```python
from build123d import *

# Parameters (mm, degrees)
SKETCH3_R           = 1.905
BOSS_EXTRUDE1_DEPTH = 6.35
CUT_EXTRUDE1_DEPTH  = 133.5410974
SKETCH5_R           = 1.905
BOSS_EXTRUDE2_DEPTH = 12.700000124
CUT_EXTRUDE2_START  = -6.350000124
SKETCH6_R           = 1.905
SKETCH6_R_2         = 1.75
CUT_EXTRUDE2_DEPTH  = 6.350000124


with BuildPart() as part:
    # Sketch3 → Boss-Extrude1 (new body)
    with BuildSketch(Plane(origin=(0, 0, 0), x_dir=(1, 0, 0), z_dir=(0, 1, 0))):
        Polygon((-19.05, -82.55), (-12.7, -88.9), (12.7, -88.9), (19.05, -82.55), (19.05, -74.93), (19.05, -68.58), (19.05, -60.96), (19.05, -38.1), (19.05, -30.48), (19.05, -24.13), (19.05, -16.51), (49.05, 15.745), (49.05, 27.745), (-49.05, 27.745), (-49.05, 15.745), (-19.05, -16.51), (-19.05, -24.13), (-19.05, -30.48), (-19.05, -38.1), (-19.05, -60.96), (-19.05, -68.58), (-19.05, -74.93), align=None)
        with Locations(Location((-15.24, -78.74, 0), (0, 0, 270))):
            Circle(SKETCH3_R, mode=Mode.SUBTRACT)
        with Locations(Location((15.24, -78.74, 0), (0, 0, 270))):
            Circle(SKETCH3_R, mode=Mode.SUBTRACT)
        with Locations(Location((15.24, -64.77, 0), (0, 0, 270))):
            Circle(SKETCH3_R, mode=Mode.SUBTRACT)
        with Locations(Location((-15.24, -64.77, 0), (0, 0, 270))):
            Circle(SKETCH3_R, mode=Mode.SUBTRACT)
        with Locations(Location((-15.24, -20.32, 0), (0, 0, 270))):
            Circle(SKETCH3_R, mode=Mode.SUBTRACT)
        with Locations(Location((15.24, -20.32, 0), (0, 0, 270))):
            Circle(SKETCH3_R, mode=Mode.SUBTRACT)
        with Locations(Location((15.24, -34.29, 0), (0, 0, 270))):
            Circle(SKETCH3_R, mode=Mode.SUBTRACT)
        with Locations(Location((-15.24, -34.29, 0), (0, 0, 270))):
            Circle(SKETCH3_R, mode=Mode.SUBTRACT)
    extrude(amount=BOSS_EXTRUDE1_DEPTH)

    # Sketch4 → Cut-Extrude1 (cut, through all)
    with BuildSketch(Plane.ZY.offset(49.05)):
        Polygon((-21.395, 0), (-27.745, 0), (-27.745, 5), align=None)
    extrude(amount=-CUT_EXTRUDE1_DEPTH, mode=Mode.SUBTRACT)

    # Sketch5 → Boss-Extrude2 (add)
    with BuildSketch(Plane.XZ):
        with Locations(Location((-15.24, 20.32, 0), (0, 0, 270))):
            Circle(SKETCH5_R)
        with Locations(Location((-15.24, 34.29, 0), (0, 0, 270))):
            Circle(SKETCH5_R)
        with Locations(Location((15.24, 20.32, 0), (0, 0, 270))):
            Circle(SKETCH5_R)
        with Locations(Location((15.24, 34.29, 0), (0, 0, 270))):
            Circle(SKETCH5_R)
        with Locations(Location((15.24, 64.77, 0), (0, 0, 270))):
            Circle(SKETCH5_R)
        with Locations(Location((15.24, 78.74, 0), (0, 0, 270))):
            Circle(SKETCH5_R)
        with Locations(Location((-15.24, 64.77, 0), (0, 0, 270))):
            Circle(SKETCH5_R)
        with Locations(Location((-15.24, 78.74, 0), (0, 0, 270))):
            Circle(SKETCH5_R)
    extrude(amount=-BOSS_EXTRUDE2_DEPTH)

    # Sketch6 → Cut-Extrude2 (cut)
    # profile 1 of 8: a face of its own
    with BuildSketch(Plane(origin=(0, 12.700000124, 0), x_dir=(1, 0, 0), z_dir=(0, 1, 0)).offset(CUT_EXTRUDE2_START)):
        with Locations((-15.24, -78.74)):
            Circle(SKETCH6_R)
        with Locations(Location((-15.24, -78.74, 0), (0, 0, 270))):
            Circle(SKETCH6_R_2, mode=Mode.SUBTRACT)
    # profile 2 of 8: a face of its own
    with BuildSketch(Plane(origin=(0, 12.700000124, 0), x_dir=(1, 0, 0), z_dir=(0, 1, 0)).offset(CUT_EXTRUDE2_START)):
        with Locations((15.24, -78.74)):
            Circle(SKETCH6_R)
        with Locations(Location((15.24, -78.74, 0), (0, 0, 270))):
            Circle(SKETCH6_R_2, mode=Mode.SUBTRACT)
    # profile 3 of 8: a face of its own
    with BuildSketch(Plane(origin=(0, 12.700000124, 0), x_dir=(1, 0, 0), z_dir=(0, 1, 0)).offset(CUT_EXTRUDE2_START)):
        with Locations((15.24, -64.77)):
            Circle(SKETCH6_R)
        with Locations(Location((15.24, -64.77, 0), (0, 0, 270))):
            Circle(SKETCH6_R_2, mode=Mode.SUBTRACT)
    # profile 4 of 8: a face of its own
    with BuildSketch(Plane(origin=(0, 12.700000124, 0), x_dir=(1, 0, 0), z_dir=(0, 1, 0)).offset(CUT_EXTRUDE2_START)):
        with Locations((-15.24, -64.77)):
            Circle(SKETCH6_R)
        with Locations(Location((-15.24, -64.77, 0), (0, 0, 270))):
            Circle(SKETCH6_R_2, mode=Mode.SUBTRACT)
    # profile 5 of 8: a face of its own
    with BuildSketch(Plane(origin=(0, 12.700000124, 0), x_dir=(1, 0, 0), z_dir=(0, 1, 0)).offset(CUT_EXTRUDE2_START)):
        with Locations((-15.24, -34.29)):
            Circle(SKETCH6_R)
        with Locations(Location((-15.24, -34.29, 0), (0, 0, 270))):
            Circle(SKETCH6_R_2, mode=Mode.SUBTRACT)
    # profile 6 of 8: a face of its own
    with BuildSketch(Plane(origin=(0, 12.700000124, 0), x_dir=(1, 0, 0), z_dir=(0, 1, 0)).offset(CUT_EXTRUDE2_START)):
        with Locations((15.24, -34.29)):
            Circle(SKETCH6_R)
        with Locations(Location((15.24, -34.29, 0), (0, 0, 270))):
            Circle(SKETCH6_R_2, mode=Mode.SUBTRACT)
    # profile 7 of 8: a face of its own
    with BuildSketch(Plane(origin=(0, 12.700000124, 0), x_dir=(1, 0, 0), z_dir=(0, 1, 0)).offset(CUT_EXTRUDE2_START)):
        with Locations((15.24, -20.32)):
            Circle(SKETCH6_R)
        with Locations(Location((15.24, -20.32, 0), (0, 0, 270))):
            Circle(SKETCH6_R_2, mode=Mode.SUBTRACT)
    # profile 8 of 8: a face of its own
    with BuildSketch(Plane(origin=(0, 12.700000124, 0), x_dir=(1, 0, 0), z_dir=(0, 1, 0)).offset(CUT_EXTRUDE2_START)):
        with Locations((-15.24, -20.32)):
            Circle(SKETCH6_R)
        with Locations(Location((-15.24, -20.32, 0), (0, 0, 270))):
            Circle(SKETCH6_R_2, mode=Mode.SUBTRACT)
    extrude(amount=CUT_EXTRUDE2_DEPTH, mode=Mode.SUBTRACT)


solid = part.part
```
For this review, take the finished solid that the model builds, in its own axes (mm). A direction names the side the tool comes from. Round coordinates to 2 decimals unless told otherwise and drop trailing zeros. Order: outer loops, then holes, each group sorted by start corner. A loop starts at its lowest first (then second) coordinate and runs counter-clockwise, first axis right, second up. Notation, with made-up numbers: (0, -26.5) -> (18, -26.5) arc R26 cw to (18, 3.5) -> close; hole circle Ø6 at (-38.5, -26.5). An arc over 180 degrees is marked (long way). Use a Markdown table: item, result.
Item 1: Draft analysis for pull direction X (two halves, no side actions). For faces 1 (the flat face through (-49.05, 4, -20)), 2 (the cylindrical face through (-15.16, 9.48, 76.99)), 3 (the flat face through (15, 12.7, 20)), state which applies: +X half, -X half, draft (parallel to the pull), parting line (faces both ways), or undercut.
Resolved:
| item | result |
|---|---|
| face 1 | -X half |
| face 2 | undercut |
| face 3 | draft |
Item 2: Take a section at D-D (z = 45). State the section outline as (x, y) points.
Resolved:
| item | result |
|---|---|
| outline | (-19.05, 0) -> (19.05, 0) -> (19.05, 6.35) -> (-19.05, 6.35) -> close |
Item 3: Take a section at B-B (z = 20.32). State the section outline as (x, y) points.
Resolved:
| item | result |
|---|---|
| outline | (-19.05, 0) -> (19.05, 0) -> (19.05, 6.35) -> (16.99, 6.35) -> (16.99, 12.7) -> (13.49, 12.7) -> (13.49, 6.35) -> (-13.49, 6.35) -> (-13.49, 12.7) -> (-16.99, 12.7) -> (-16.99, 6.35) -> (-19.05, 6.35) -> close |
Item 4: Machinability: for faces 4 (the flat face through (-15, 12.7, 34)), 5 (the flat face through (19.05, 3, 50)), 6 (the cylindrical face through (14.6, 9.5, 66.4)), which of the approach directions +Z, -Z, +X, -X, +Y, -Y give a long, thin tool a straight path to every point of the face, cutting with its end or side? Answer none if there is none.
Resolved:
| item | result |
|---|---|
| face 4 | +Z, -Z, +X, -X, +Y |
| face 5 | +Z, +X, +Y, -Y |
| face 6 | +Y |
Item 5: Take a section at A-A (x = -15.24). State the section outline as (y, z) points (3 decimals), plus the area to 3 significant figures.
Resolved:
| item | result |
|---|---|
| outline | (0, -21.395) -> (5, -27.745) -> (6.35, -27.745) -> (6.35, 18.57) -> (12.7, 18.57) -> (12.7, 22.07) -> (6.35, 22.07) -> (6.35, 32.54) -> (12.7, 32.54) -> (12.7, 36.04) -> (6.35, 36.04) -> (6.35, 63.02) -> (12.7, 63.02) -> (12.7, 66.52) -> (6.35, 66.52) -> (6.35, 76.99) -> (12.7, 76.99) -> (12.7, 80.49) -> (6.35, 80.49) -> (6.35, 86.36) -> (0, 86.36) -> close |
| area | 798 mm² |
Item 6: For pin 1 (4 mm diameter, centred on y = 7.5, z = 74, fed in from -X); pin 2 (12 mm diameter, centred on x = 24.5, z = -9, fed in from +Y); pin 3 (1.9 mm diameter, centred on y = 4.5, z = 53.5, fed in from +X), all flat-tipped, find the tip position at first contact; note any pin that passes through.
Resolved:
| item | result |
|---|---|
| pin 1 | stops at x = -19.05 |
| pin 2 | stops at y = 6.35 |
| pin 3 | stops at x = 19.05 |
Item 7: For line 1 along Y through (x, z) = (10, -6); line 2 along X through (y, z) = (4.25, 40.5); line 3 along X through (y, z) = (7.5, 19), list the stretches that pass through material, from the lowest coordinate up. Write a range as [from, to].
Resolved:
| item | result |
|---|---|
| line 1 | y = [0, 6.35] |
| line 2 | x = [-19.05, 19.05] |
| line 3 | x = [-16.39, -14.09], [14.09, 16.39] |
Item 8: Take a section at C-C (x = -25.5). State the section outline as (y, z) points (3 decimals).
Resolved:
| item | result |
|---|---|
| outline | (0, -21.395) -> (5, -27.745) -> (6.35, -27.745) -> (6.35, 9.575) -> (0, 9.575) -> close |
